Work out the finished part from the listing and answer in its coordinate system (mm). A direction names the side the tool comes from. Round coordinates to 2 decimals unless told otherwise and drop trailing zeros. Order: outer loops, then holes, each group sorted by start corner. A loop starts at its lowest first (then second) coordinate and runs counter-clockwise, first axis right, second up. Notation, with made-up numbers: M 13,18.5 L 69,18.5 A19 cw 69,44.5 Z; hole C -10.5,78.25 d1. An arc over 180 degrees is marked long. Return JSON: item names as keys, results as strings.
from build123d import *

# Parameters (mm, degrees)
SKETCH_1_R      = 6
EXTRUDE_1_DEPTH = 12
SKETCH_2_R      = 2.5
EXTRUDE_2_DEPTH = 30
CHAMFER_1_SIZE  = 1


with BuildPart() as part:
    # Эскиз1 → Вытянуть1 (new body)
    with BuildSketch(Plane(origin=(0, 0, 0), x_dir=(1, 0, 0), z_dir=(0, 1, 0))):
        with Locations(Location((0, 0, 0), (0, 0, 270))):
            Circle(SKETCH_1_R)
    extrude(amount=EXTRUDE_1_DEPTH)

    # Эскиз2 → Вытянуть2 (add)
    with BuildSketch(Plane(origin=(0, 12, 0), x_dir=(1, 0, 0), z_dir=(0, 1, 0))):
        with Locations(Location((0, 0, 0), (0, 0, 270))):
            Circle(SKETCH_2_R)
    extrude(amount=EXTRUDE_2_DEPTH)

    # Фаска1
    chamfer_1_edges = [part.edges().sort_by_distance(p)[0] for p in [
        (0, 12, -6),
        (0, 42, -2.5),
    ]]
    chamfer(chamfer_1_edges, length=CHAMFER_1_SIZE)


solid = part.part
Item 1: Which of the six approach directions +Z, -Z, +X, -X, +Y, -Y give full straight-line access (tool end or side, diameter ignored) to faces 1 (the flat face through (-2, 12, 2)), 2 (the flat face through (0, 42, 0))?
Output:
{"face 1": "+Y", "face 2": "+Z, -Z, +X, -X, +Y"}
Item 2: Find section D-D (y = 7.5). Determine the outline of the cut face in (x, z), plus the area to 3 significant figures.
Output:
{"outline": "C 0,0 d12", "area": "113 mm^2"}
Item 3: Each of these flat-tipped pins is pushed along its axis until it touches: pin 1 (5 mm diameter, centred on x = -2, y = 25, fed in from -Z); pin 2 (1 mm diameter, centred on x = 0.5, y = 16, fed in from +Z); pin 3 (4 mm diameter, centred on y = 36.5, z = 4, fed in from +X). Where does it stop, or does it pass through?
Output:
{"pin 1": "stops at z = -2.5", "pin 2": "stops at z = 2.5", "pin 3": "stops at x = 1.5"}
Item 4: Find section C-C (y = 21). Determine the outline of the cut face in (x, z), plus the area to 3 significant figures.
Output:
{"outline": "C 0,0 d5", "area": "19.6 mm^2"}
Item 5: Find section B-B (z = 0). Determine the outline of the cut face in (x, y).
Output:
{"outline": "M -6,0 L 6,0 L 6,11 L 5,12 L 2.5,12 L 2.5,41 L 1.5,42 L -1.5,42 L -2.5,41 L -2.5,12 L -5,12 L -6,11 Z"}
Item 6: Find section A-A (x = 0). Determine the outline of the cut face in (y, z).
Output:
{"outline": "M 0,-6 L 11,-6 L 12,-5 L 12,-2.5 L 41,-2.5 L 42,-1.5 L 42,1.5 L 41,2.5 L 12,2.5 L 12,5 L 11,6 L 0,6 Z"}
Item 7: Consider line 1 along Y through (x, z) = (-2.5, 2.5); line 2 along X through (y, z) = (9.5, -0.25); line 3 along X through (y, z) = (17.5, -0.5). Determine where each line is inside the solid, lowest interval first. Write a range as [from, to].
Output:
{"line 1": "y = [0, 12]", "line 2": "x = [-5.99, 5.99]", "line 3": "x = [-2.45, 2.45]"}
